Input: dimensioned drawing with shaded views. Units: mm. Origin: part minimum x, y, z. Round coordinates to 2 decimals unless told otherwise and drop trailing zeros. Order: outer loops, then holes, each group sorted by start corner. A loop starts at its lowest first (then second) coordinate and runs counter-clockwise, first axis right, second up. Notation, with made-up numbers: (-7.75, -37) - (17.25, -37) arc R23 cw to (17.25, -6) - close; hole circle Ø11 at (51, 23). An arc over 180 degrees is marked (long way). One line per item, written item: value. Start each with the question number.
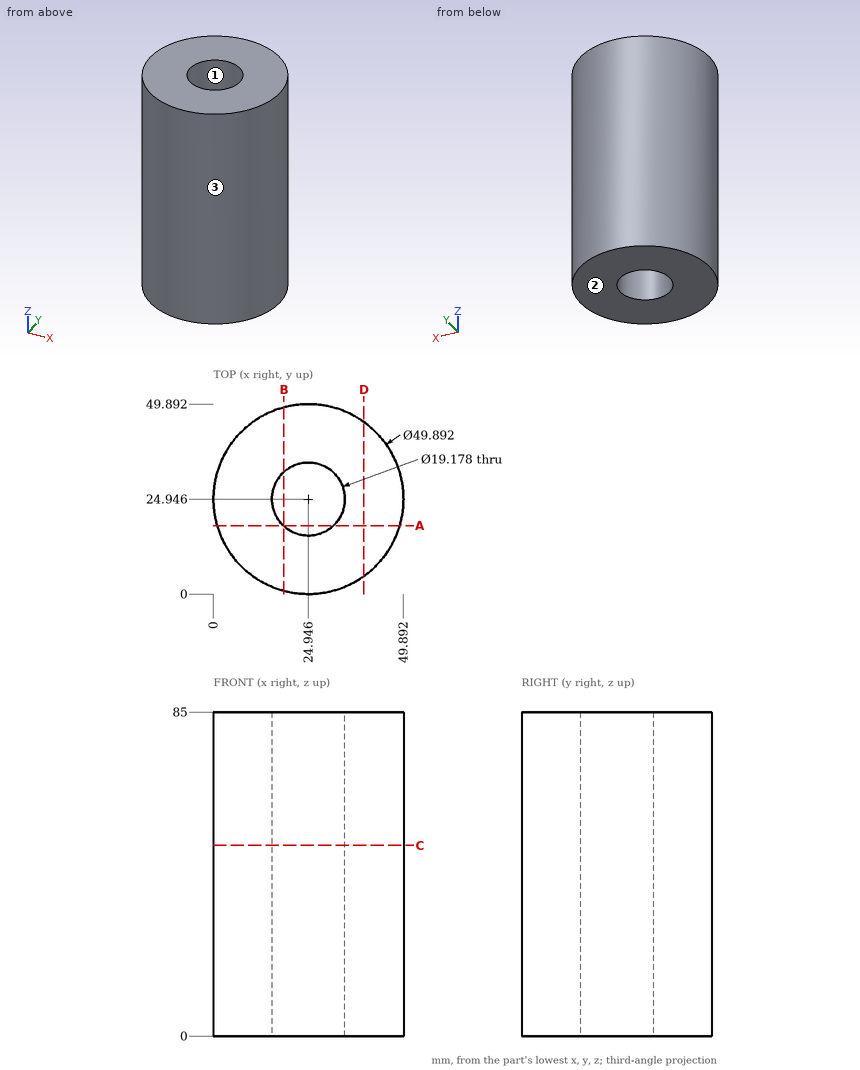
1. Section D-D (x = 39.5). Return the cut outline in (y, z), then the cut area to 3 significant figures.
2. Section C-C (z = 50). Return the cut outline in (x, y) (3 decimals), then the cut area to 3 significant figures.
3. Pin query (flat end, axial travel): pin 1 (5 mm diameter, centred on x = 36.5, z = 65, fed in from +Y); pin 2 (2 mm diameter, centred on y = 42.5, z = 25.5, fed in from +X); pin 3 (6 mm diameter, centred on x = 23, y = 19.5, fed in from +Z); pin 4 (12 mm diameter, centred on y = 7, z = 33, fed in from +X). Return the tip coordinate at first contact, or that it passes through.
4. Section A-A (y = 18). Return the cut outline in (x, z).
5. Section B-B (x = 18.5). Return the cut outline in (y, z), then the cut area to 3 significant figures.
6. Line query: line 1 (Y direction, x = 25, z = 56) (3 decimals); line 2 (X direction, y = 20, z = 65.5) (3 decimals); line 3 (Y direction, x = 20.5, z = 68). Output: solid intervals per line, ascending. Write a range as from..to.
7. Pull-direction query (Y, two-part tool) for the marked faces 1, 2 and 3; classes: released by +Y, released by -Y, zero draft, split by the parting line, or undercut.
Solved:
1. outline: (4.69, 0) - (45.21, 0) - (45.21, 85) - (4.69, 85) - close
1. area: 3,440 mm²
2. outline: circle Ø49.892 at (24.946, 24.946); hole circle Ø19.178 at (24.946, 24.946)
2. area: 1,670 mm²
3. pin 1: stops at y = 48.19
3. pin 2: stops at x = 43.61
3. pin 3: passes through
3. pin 4: stops at x = 46.85
4. outline: (0.99, 0) - (18.34, 0) - (18.34, 85) - (0.99, 85) - close; (31.56, 0) - (48.91, 0) - (48.91, 85) - (31.56, 85) - close
5. outline: (0.85, 0) - (17.85, 0) - (17.85, 85) - (0.85, 85) - close; (32.05, 0) - (49.04, 0) - (49.04, 85) - (32.05, 85) - close
5. area: 2,890 mm²
6. line 1: y = 0..15.357, 34.535..49.892
6. line 2: x = 0.495..16.731, 33.161..49.397
6. line 3: y = 0.4..16.45, 33.44..49.49
7. face 1: undercut
7. face 2: zero draft
7. face 3: split by the parting line
